Here's how the part is built. I have some questions about the finished solid (model axes, mm). A direction names the side the tool comes from. Give positions to 0.01 mm unless a question says otherwise; leave off trailing zeros. Order: outer loops, then holes, each group sorted by start corner. A loop starts at its lowest first (then second) coordinate and runs counter-clockwise, first axis right, second up. Notation, with made-up numbers: (1, 68.25) -> (32, 68.25) arc R13 ccw to (32, 73.25) -> close; hole circle Ø3 at (19.25, 83). An arc over 180 degrees is marked (long way). Write each question's results on one line, items separated by ' | '. Start each with the question number.
Q1. Imagine slicing it at B-B, the plane x = 22.5. Please give me the cut outline in (y, z).
Q2. Imagine slicing it at D-D, the plane y = 11. Please give me the cut outline in (x, z).
Q3. I need wall thicknesses on line 1 along X through (y, z) = (7, 1.5); line 2 along Y through (x, z) = (7.5, 1.7); line 3 along Z through (x, y) = (15.75, 1.75). Which ranges of each line are inside material? Lowest first, please. Write a range as [from, to].
Q4. I'm going to push flat-ended pins straight in: pin 1 (0.8 mm diameter, centred on y = 12, z = 5.5, fed in from +X); pin 2 (0.5 mm diameter, centred on x = 18.5, z = 5.5, fed in from +Y); pin 3 (0.5 mm diameter, centred on y = 7.5, z = 5.5, fed in from -X); pin 4 (1.1 mm diameter, centred on x = 27, z = 5.5, fed in from +Y). Where does each tip first touch, or does it pass through?
Q5. Imagine slicing it at C-C, the plane z = 4.5. Please give me the cut outline in (x, y).
Q6. For faces 1 (the face through (27.2, 9.1, 5.5)), 2 (the face through (27.2, 5.9, 5.5)), 3 (the face through (15, 8, 5)), 4 (the face through (9.1, 12.2, 5.5)), which set-ups out of +Z, -Z, +X, -X, +Y, -Y let a thin tool reach every point of the face, with its end or its side?
Q7. Thinking about a two-plate mould opening in Y: for faces 5 (the face through (7.5, 9.5, 5.5)), 6 (the face through (24.5, 7.5, 5.5)), 7 (the face through (0.285, 14.699, 2.732)), 8 (the face through (7.15, 5.94, 2.67)), which applies, pulls with the +Y half, pulls with the -Y half, needs draft (parallel to the pull), parting line crosses it, or undercut?
Q8. Imagine slicing it at A-A, the plane y = 7.5. Please give me the cut outline in (x, z), then the cut area to 3 significant figures.
```python
from build123d import *

# Parameters (mm, degrees)
SKETCH039_W                                      = 30
SKETCH039_H                                      = 15
SKETCH039_R                                      = 1.6
PAD008_DEPTH                                     = 5
SKETCH040_W                                      = 4.5
SKETCH040_H                                      = 3.2
SKETCH040_W_2                                    = 5.5
SKETCH040_W_3                                    = 3.2
SKETCH040_H_2                                    = 5.5
PAD009_DEPTH                                     = 1
PAD010_DEPTH                                     = 1
FILLET002_R                                      = 1
CHAMFER004013007011015006009007001005003045_SIZE = 0.4
CHAMFER004013007011015006009007001005003046_SIZE = 0.4


with BuildPart() as part:
    # Sketch039 → Pad008 (new body)
    with BuildSketch(Plane.XY):
        with Locations((15, 7.5)):
            Rectangle(SKETCH039_W, SKETCH039_H)
        with Locations((7.5, 7.5)):
            Circle(SKETCH039_R, mode=Mode.SUBTRACT)
        with Locations((22.5, 7.5)):
            Circle(SKETCH039_R, mode=Mode.SUBTRACT)
    extrude(amount=PAD008_DEPTH)

    # Sketch040 (on Face8 of Pad008) → Pad009 (join)
    with BuildSketch(Plane.XY.offset(5)):
        with Locations((18.25, 7.5)):
            Rectangle(SKETCH040_W, SKETCH040_H)
        with Locations((27.25, 7.5)):
            Rectangle(SKETCH040_W_2, SKETCH040_H)
        with Locations((7.5, 12.25)):
            Rectangle(SKETCH040_W_3, SKETCH040_H_2)
        with Locations((7.5, 2.75)):
            Rectangle(SKETCH040_W_3, SKETCH040_H_2)
    extrude(amount=PAD009_DEPTH)

    # Sketch040 (on Face8 of Pad008) → Pad010 (join)
    with BuildSketch(Plane.XY.offset(5)):
        with Locations((18.25, 7.5)):
            Rectangle(SKETCH040_W, SKETCH040_H)
        with Locations((27.25, 7.5)):
            Rectangle(SKETCH040_W_2, SKETCH040_H)
        with Locations((7.5, 12.25)):
            Rectangle(SKETCH040_W_3, SKETCH040_H_2)
        with Locations((7.5, 2.75)):
            Rectangle(SKETCH040_W_3, SKETCH040_H_2)
    extrude(amount=PAD010_DEPTH)

    # Fillet002
    fillet002_edges = [part.edges().sort_by_distance(p)[0] for p in [
        (30, 0, 2.5),
        (30, 15, 2.5),
        (0, 15, 2.5),
        (0, 0, 2.5),
    ]]
    fillet(fillet002_edges, radius=FILLET002_R)

    # Chamfer004013007011015006009007001005003045
    chamfer004013007011015006009007001005003045_edges = [part.edges().sort_by_distance(p)[0] for p in [
        (30, 9.1, 5.5),
        (24.5, 9.1, 5.5),
        (20.5, 9.1, 5.5),
        (16, 9.1, 5.5),
        (16, 5.9, 5.5),
        (9.1, 15, 5.5),
        (5.9, 15, 5.5),
        (9.1, 5.5, 5.5),
        (5.9, 5.5, 5.5),
        (5.9, 9.5, 5.5),
        (5.9, 0, 5.5),
        (9.1, 9.5, 5.5),
        (9.1, 0, 5.5),
        (20.5, 5.9, 5.5),
        (24.5, 5.9, 5.5),
        (30, 5.9, 5.5),
    ]]
    chamfer(chamfer004013007011015006009007001005003045_edges, length=CHAMFER004013007011015006009007001005003045_SIZE)

    # Chamfer004013007011015006009007001005003046
    chamfer004013007011015006009007001005003046_edges = [part.edges().sort_by_distance(p)[0] for p in [
        (15, 0, 0),
        (29.707107, 0.292893, 0),
        (30, 7.5, 0),
        (29.707107, 14.707107, 0),
        (15, 15, 0),
        (0.292893, 14.707107, 0),
        (0, 7.5, 0),
        (0.292893, 0.292893, 0),
        (20.9, 7.5, 0),
        (5.9, 7.5, 0),
    ]]
    chamfer(chamfer004013007011015006009007001005003046_edges, length=CHAMFER004013007011015006009007001005003046_SIZE)


solid = part.part
```
Geometry check:
1) outline: (0, 0.4) -> (0.4, 0) -> (5.5, 0) -> (5.9, 0.4) -> (5.9, 5) -> (0, 5) -> close; (9.1, 0.4) -> (9.5, 0) -> (14.6, 0) -> (15, 0.4) -> (15, 5) -> (9.1, 5) -> close
2) outline: (0, 0.4) -> (0.4, 0) -> (29.6, 0) -> (30, 0.4) -> (30, 5) -> (9.1, 5) -> (9.1, 6) -> (5.9, 6) -> (5.9, 5) -> (0, 5) -> close
3) line 1: [0, 5.98], [9.02, 20.98], [24.02, 30] | line 2: [0, 5.9], [9.1, 15] | line 3: [0, 5]
4) pin 1: x = 9.1 | pin 2: y = 9.1 | pin 3: x = 16 | pin 4: y = 15
5) outline: (0, 1) arc R1 ccw to (1, 0) -> (29, 0) arc R1 ccw to (30, 1) -> (30, 14) arc R1 ccw to (29, 15) -> (1, 15) arc R1 ccw to (0, 14) -> close; hole circle Ø3.2 at (7.5, 7.5); hole circle Ø3.2 at (22.5, 7.5)
6) face 1: +Z, +X, -X, +Y | face 2: +Z, +X, -X, -Y | face 3: +Z | face 4: +Z, +X, +Y, -Y
7) face 5: undercut | face 6: needs draft | face 7: pulls with the +Y half | face 8: undercut
8) outline: (0, 0.4) -> (0.4, 0) -> (5.5, 0) -> (5.9, 0.4) -> (5.9, 5) -> (0, 5) -> close; (9.1, 0.4) -> (9.5, 0) -> (20.5, 0) -> (20.9, 0.4) -> (20.9, 5) -> (20.5, 5) -> (20.5, 6) -> (16, 6) -> (16, 5) -> (9.1, 5) -> close; (24.1, 0.4) -> (24.5, 0) -> (29.6, 0) -> (30, 0.4) -> (30, 6) -> (24.5, 6) -> (24.5, 5) -> (24.1, 5) -> close | area: 128 mm²
